Geometry check sheet. Reference: the model listing, model coordinates, mm. A direction names the side the tool comes from. Round coordinates to 2 decimals unless told otherwise and drop trailing zeros. Loops run counter-clockwise (first coordinate to the right, second up) from the corner with the lowest first, then second, coordinate; pieces in that order, holes last. Notation, with made-up numbers: (36.5, 72) -> (63.5, 72) arc R13 cw to (63.5, 80) -> close; hole circle Ø9 at (-23.5, 12.25). An arc over 180 degrees is marked (long way). Use a Markdown table: item, result. Add a question column.
Q1. Sectioned sample at C-C, the plane z = 5. Enter the section's corners in (x, y), then the cut area to 3 significant figures.
Q2. Material ranges on L1, parallel to Z at x = 5.75, y = 16; L2, parallel to Z at x = 4.25, y = 24.5, recorded low to high.
Q3. Gauge pin test, flat ends, axial feed: P1, Ø4, axis at y = 22.5, z = 0.5, coming from the +X side; P2, Ø0.8, axis at x = 4, y = 22, coming from the -Z side; P3, Ø12, axis at y = 9.5, z = -3.5, coming from the -X side; P4, Ø2.5, axis at y = 11.5, z = -2.5, coming from the +X side. Record the tip position at first contact, or that the pin passes through.
Q4. Set-up check for faces 5 (the face through (4.92, 18.73, 5.98)), 6 (the face through (4, 19, -8.5)), 7 (the face through (9.3, 18.7, 3.8)), 8 (the face through (-7, 19, -10)), 9 (the face through (-3.7, 18.7, -9.2)): record each of +Z, -Z, +X, -X, +Y, -Y from which the full face is reachable in a straight line by a thin tool's end or side.
Q5. Sectioned sample at A-A, the plane z = -5. Enter the section's corners in (x, y), then the cut area to 3 significant figures.
Q6. Release check for a two-part mould opening along X. For faces 1 (the face through (-9.3, 18.7, -3.8)), 2 (the face through (2, 19, -4.5)), 3 (the face through (9.2, 18.7, -3.7)), 4 (the face through (3, 38, -2)) record: released by +X, released by -X, zero draft, split by the parting line, or undercut.
Q7. Sectioned sample at B-B, the plane x = -1.5. Enter the section's corners in (y, z), then the cut area to 3 significant figures.
```python
from build123d import *

# Parameters (mm, degrees)
ESQUISSE1_R      = 2.5
EXTRUSION1_DEPTH = 38
CONG_1_R         = 0.75
EXTRUSION2_REACH = 40


with BuildPart() as part:
    # Esquisse1 → Extrusion1 (new body)
    with BuildSketch(Plane(origin=(0, 0, 0), x_dir=(1, 0, 0), z_dir=(0, 1, 0))):
        Polygon((0, 4), (-0.5, 4.5), (-3.439339828, 4.5), (-6.439339828, 7.5), (-6.439339828, 8.5), (-3, 8.5), (-4.5, 10), (-10, 10), (-10, 4.5), (-8.5, 3), (-8.5, 6.439339828), (-7.5, 6.439339828), (-4.5, 3.439339828), (-4.5, 0.5), (-4, 0), (-4.5, -0.5), (-4.5, -3.439339828), (-7.5, -6.439339828), (-8.5, -6.439339828), (-8.5, -3), (-10, -4.5), (-10, -10), (-4.5, -10), (-3, -8.5), (-6.439339828, -8.5), (-6.439339828, -7.5), (-3.439339828, -4.5), (-0.5, -4.5), (0, -4), (0.5, -4.5), (3.439339828, -4.5), (6.439339828, -7.5), (6.439339828, -8.5), (3, -8.5), (4.5, -10), (10, -10), (10, -4.5), (8.5, -3), (8.5, -6.439339828), (7.5, -6.439339828), (4.5, -3.439339828), (4.5, -0.5), (4, 0), (4.5, 0.5), (4.5, 3.439339828), (7.5, 6.439339828), (8.5, 6.439339828), (8.5, 3), (10, 4.5), (10, 10), (4.5, 10), (3, 8.5), (6.439339828, 8.5), (6.439339828, 7.5), (3.439339828, 4.5), (0.5, 4.5), align=None)
        Circle(ESQUISSE1_R, mode=Mode.SUBTRACT)
    extrude(amount=EXTRUSION1_DEPTH)

    # Congé1
    cong_1_edges = [part.edges().sort_by_distance(p)[0] for p in [
        (6.439339828, 19, -8.5),
        (10, 19, -10),
        (8.5, 19, -6.439339828),
        (8.5, 19, 6.439339828),
        (10, 19, 10),
        (6.439339828, 19, 8.5),
        (-6.439339828, 19, 8.5),
        (-10, 19, 10),
        (-8.5, 19, 6.439339828),
        (-8.5, 19, -6.439339828),
        (-10, 19, -10),
        (-6.439339828, 19, -8.5),
    ]]
    fillet(cong_1_edges, radius=CONG_1_R)

    # Esquisse2 → Extrusion2 (cut, up to next)
    with BuildSketch(Plane(origin=(0, 38, 0), x_dir=(1, 0, 0), z_dir=(0, 1, 0)), mode=Mode.PRIVATE) as extrusion2_sk1:
        Polygon((-3.439339828, -4.5), (-4.5, -3.439339828), (-8.5, -3), (-10, -4.5), (-10, -10), (-4.5, -10), (-3, -8.5), align=None)
    extrusion2_tool1 = extrude(extrusion2_sk1.sketch, amount=-EXTRUSION2_REACH, mode=Mode.PRIVATE) & part.part
    add(extrusion2_tool1.solids().sort_by_distance((-6.693883, 38, 6.693883))[0], mode=Mode.SUBTRACT)


solid = part.part
```
Values:
| question | item | result |
|---|---|---|
| 1 | outline | (3.94, 0) -> (6.06, 0) -> (6.06, 38) -> (3.94, 38) -> close; (8.5, 0) -> (10, 0) -> (10, 38) -> (8.5, 38) -> close |
| 1 | area | 138 mm^2 |
| 2 | L1 | -10 to -8.5, -6.81 to -4.69, 4.69 to 6.81, 8.5 to 10 |
| 2 | L2 | -9.75 to -8.5, -5.31 to -0.25, 0.25 to 5.31, 8.5 to 9.75 |
| 3 | P1 | x = 4.5 |
| 3 | P2 | z = -9.9 |
| 3 | P3 | x = -10 |
| 3 | P4 | x = 9.25 |
| 4 | face 5 | -X, +Y, -Y |
| 4 | face 6 | +Y, -Y |
| 4 | face 7 | +X, +Y, -Y |
| 4 | face 8 | -Z, +X, -X, +Y, -Y |
| 4 | face 9 | -Z, +Y, -Y |
| 5 | outline | (-10, 0) -> (-8.5, 0) -> (-8.5, 38) -> (-10, 38) -> close; (-6.06, 0) -> (-3.94, 0) -> (-3.94, 38) -> (-6.06, 38) -> close; (3.94, 0) -> (6.06, 0) -> (6.06, 38) -> (3.94, 38) -> close; (8.5, 0) -> (10, 0) -> (10, 38) -> (8.5, 38) -> close |
| 5 | area | 275 mm^2 |
| 6 | face 1 | released by -X |
| 6 | face 2 | undercut |
| 6 | face 3 | released by +X |
| 6 | face 4 | zero draft |
| 7 | outline | (0, -4.5) -> (38, -4.5) -> (38, -2) -> (0, -2) -> close; (0, 2) -> (38, 2) -> (38, 4.5) -> (0, 4.5) -> close |
| 7 | area | 190 mm^2 |
